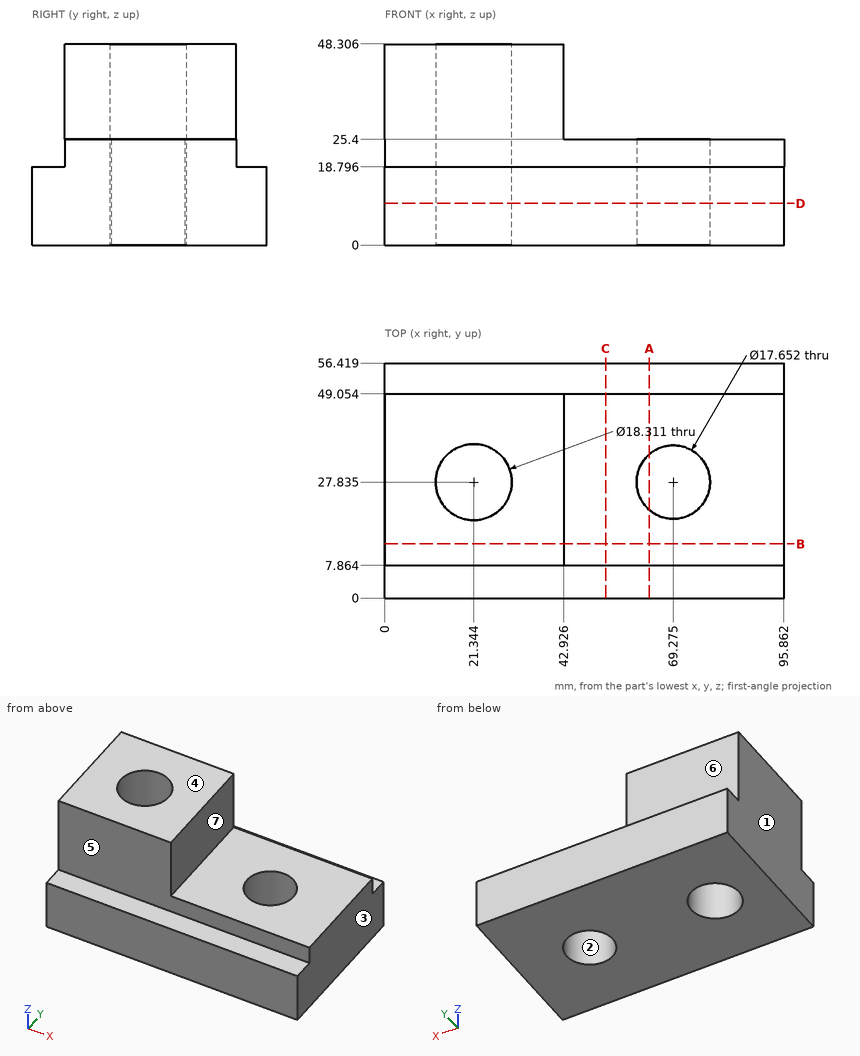
Print and shaded views of the part. All mm, measured from the part's lowest x, y and z. A direction names the side the tool comes from. Round coordinates to 2 decimals unless told otherwise and drop trailing zeros. Write each loop counter-clockwise with the first axis right and the second up, starting at its lowest first coordinate (ties: lowest second). Pieces come first, ordered by that corner, then holes. Notation, with made-up numbers: (58, 45) - (84, 45) arc R31 cw to (84, 72) - close; hole circle Ø6 at (-2.75, -37.5). An arc over 180 degrees is marked (long way). One line per item, written item: value.
(1) Cut at B-B, the plane y = 13. Give the cut face in (x, z) (1 decimal), plus the area to 3 significant figures.
Values follow:
outline: (0, 0) - (95.9, 0) - (95.9, 25.4) - (42.9, 25.4) - (42.9, 48.3) - (0, 48.3) - close
area: 3,420 mm²
(2) Cut at A-A, the plane x = 63.5. Give the cut face in (y, z) (1 decimal).
Values follow:
outline: (0, 0) - (21.2, 0) - (21.2, 25.4) - (7.9, 25.4) - (7.9, 18.8) - (0, 18.8) - close; (34.5, 0) - (56.4, 0) - (56.4, 18.8) - (49.1, 18.8) - (49.1, 25.4) - (34.5, 25.4) - close
(3) Two-plate mould, pull along X, no slides. Class the marked faces 1, 2, 3 and 4: pulls with the +X half, pulls with the -X half, needs draft (parallel to the pull), parting line crosses it, or undercut.
Values follow:
face 1: pulls with the -X half
face 2: undercut
face 3: pulls with the +X half
face 4: needs draft
(4) Cut at D-D, the plane z = 10. Give the cut face in (x, y) (1 decimal), plus the area to 3 significant figures.
Values follow:
outline: (0, 0) - (95.9, 0) - (95.9, 56.4) - (0, 56.4) - close; hole circle Ø18.3 at (21.3, 27.8); hole circle Ø17.7 at (69.3, 27.8)
area: 4,900 mm²
(5) 3-axis set-ups, long thin cutter, end or side, ignore diameter. For the marked faces 5, 6 and 7: which of +Z, -Z, +X, -X, +Y, -Y reach the whole face in a straight line?
Values follow:
face 5: +Z, +X, -X, -Y
face 6: +Z, +X, -X, +Y
face 7: +Z, +X, +Y, -Y
(6) Drop flat-ended pins along their axis: P1, Ø4, axis at x = 60.5, y = 49.5, coming from the +Z side; P2, Ø2, axis at y = 33.5, z = 42, coming from the +X side; P3, Ø6, axis at x = 65, y = 54, coming from the +Z side; P4, Ø16.5, axis at x = 21.34, y = 27.83, coming from the -Z side. Give the stop position or say it passes through.
Values follow:
P1: stops at z = 25.4
P2: stops at x = 42.93
P3: stops at z = 18.8
P4: passes through
(7) Wall check: probe 1 along X at (y, z) = (29, 14.5) (1 decimal); probe 2 along Z at (x, y) = (44, 3.5); probe 3 along Z at (x, y) = (51.5, 13.5). Give the ranges that are in metal, low to high.
Values follow:
probe 1: x = 0 to 12.3, 30.4 to 60.5, 78 to 95.9
probe 2: z = 0 to 18.8
probe 3: z = 0 to 25.4
(8) Cut at C-C, the plane x = 53. Give the cut face in (y, z) (1 decimal), plus the area to 3 significant figures.
Values follow:
outline: (0, 0) - (56.4, 0) - (56.4, 18.8) - (49.1, 18.8) - (49.1, 25.4) - (7.9, 25.4) - (7.9, 18.8) - (0, 18.8) - close
area: 1,330 mm²
